Can you work these out from the model? Positions are in its coordinate system, mm. A direction names the side the tool comes from. Coordinates: 2 decimals unless noted, no trailing zeros. Loops run counter-clockwise (first coordinate to the right, second up) from the corner with the lowest first, then second, coordinate; pieces in that order, holes last.
```python
from build123d import *

# Parameters (mm, degrees)
F0_R     = 15
F1_DEPTH = 15
F3_DEPTH = 25
F4_R     = 5


with BuildPart() as f1:
    # F0 (on Top) → F1 (new body)
    with BuildSketch(Plane.XY):
        Circle(F0_R)
    extrude(amount=F1_DEPTH)

    # F2 (on face) → F3 (cut)
    with BuildSketch(Plane(origin=(0, 0, 0), x_dir=(1, 0, 0), z_dir=(0, 0, -1))):
        with BuildLine():
            Line((1.75, -2.12132), (1.75, 2.12132))
            ThreePointArc((1.75, 2.12132), (-2.75, 0), (1.75, -2.12132))
        make_face()
    extrude(amount=-F3_DEPTH, mode=Mode.SUBTRACT)

    # F4
    f4_edges = [f1.edges().sort_by_distance(p)[0] for p in [
        (-15, 0, 15),
    ]]
    fillet(f4_edges, radius=F4_R)


solid = f1.part
```
(1) I want a section at C-C on z = 2.5. Write out the boundary of the cut face in (x, y), then the cut area to 3 significant figures.
Check values:
outline: circle Ø30 at (0, 0); hole (1.75, -2.12) - (1.75, 2.12) arc R2.75 ccw (long way) to start
area: 686 mm2
(2) I want a section at B-B on x = 0. Write out the boundary of the cut face in (y, z), then the cut area to 3 significant figures.
Check values:
outline: (-15, 0) - (-2.75, 0) - (-2.75, 15) - (-10, 15) arc R5 ccw to (-15, 10) - close; (2.75, 0) - (15, 0) - (15, 10) arc R5 ccw to (10, 15) - (2.75, 15) - close
area: 357 mm2
(3) I'm going to push flat-ended pins straight in: pin 1 (4 mm diameter, centred on x = 5, z = 10, fed in from -Y); pin 2 (10 mm diameter, centred on x = -10, y = -11.5, fed in from +Z); pin 3 (6 mm diameter, centred on y = 11.5, z = 8.5, fed in from +X); pin 4 (1.3 mm diameter, centred on y = -0.5, z = 10.5, fed in from -X). Where does each tip first touch, or does it pass through?
Check values:
pin 1: stops at y = -14.7
pin 2: stops at z = 14.99
pin 3: stops at x = 12.36
pin 4: stops at x = -15
(4) Which directions (+Z, -Z, +X, -X, +Y, -Y) give clear straight access to the entire face, cutting with the end or side of a thin tool? Please do faces 1 (the flat face through (2, 0, 15)), 2 (the flat face through (1.75, 0, 7)).
Check values:
face 1: +Z, +X, -X, +Y, -Y
face 2: +Z, -Z
(5) If I drill on probe 1 along Y at (x, z) = (0, 3); probe 2 along Z at (x, y) = (-5, 9); probe 3 along Y at (x, z) = (0, 11.75), over which ranges is the centre line in solid material (lowest first)?
Check values:
probe 1: y = -15 to -2.75, 2.75 to 15
probe 2: z = 0 to 14.99
probe 3: y = -14.68 to -2.75, 2.75 to 14.68
(6) If we mould it in two halves opening along Y, with no side actions, what happens to faces 3 (the cylindrical face through (-14.985, 0.66, 4.93)), 4 (the flat face through (3, 0, 0)), 5 (the cylindrical face through (-2.75, -0.09, 7.4))? For each: released by +Y, released by -Y, zero draft, split by the parting line, or undercut.
Check values:
face 3: split by the parting line
face 4: zero draft
face 5: undercut
(7) I want a section at D-D on z = 10.75. Write out the boundary of the cut face in (x, y), then the cut area to 3 significant figures.
Check values:
outline: circle Ø29.89 at (0, 0); hole (1.75, -2.12) - (1.75, 2.12) arc R2.75 ccw (long way) to start
area: 681 mm2
(8) I want a section at A-A on y = 0. Write out the boundary of the cut face in (x, z).
Check values:
outline: (-15, 0) - (-2.75, 0) - (-2.75, 15) - (-10, 15) arc R5 ccw to (-15, 10) - close; (1.75, 0) - (15, 0) - (15, 10) arc R5 ccw to (10, 15) - (1.75, 15) - close
